Could you check a few things on this model? Use its own coordinates, in mm. Face numbers are marked on the shaded views. A direction names the side the tool comes from. Give positions to 0.01 mm unless a question says otherwise; leave off trailing zeros. Order: outer loops, then holes, each group sorted by start corner. A loop starts at its lowest first (then second) coordinate and runs counter-clockwise, first axis right, second up.
from build123d import *

# Parameters (mm, degrees)
SKETCH1_W           = 18
SKETCH1_H           = 14.75
BOSS_EXTRUDE1_DEPTH = 60
CUT_EXTRUDE1_REACH  = 123.108
SKETCH2_W           = 40
SKETCH2_H           = 14.75
CUT_EXTRUDE2_REACH  = 115.987
CUT_EXTRUDE3_REACH  = 123.108
SKETCH5_R           = 3.25
CUT_EXTRUDE4_REACH  = 105.817
SKETCH6_R           = 2.6
SKETCH7_R           = 2.6
CUT_EXTRUDE5_DEPTH  = 114.9871155
CUT_EXTRUDE6_REACH  = 115.987
SKETCH8_R           = 3.25
SKETCH9_W           = 23
SKETCH9_H           = 21.27
SKETCH9_H_2         = 20
CUT_EXTRUDE7_DEPTH  = 12
CHAMFER1_SIZE       = 1
CUT_EXTRUDE8_REACH  = 123.108
SKETCH10_R          = 3.1
SKETCH10_R_2        = 2.6
SKETCH11_R          = 3.25
CUT_EXTRUDE9_DEPTH  = 125.185596991
CHAMFER2_SIZE       = 1


with BuildPart() as part:
    # Sketch1 → Boss-Extrude1 (new body)
    with BuildSketch(Plane.XY):
        Polygon((0, 0), (-29, 0), (-29, 5), (-5, 5), (-5, 38), (-28, 38), (-28, 63.75), (-5, 63.75), (-5, 75.75), (18, 75.75), (18, 63.75), (73, 63.75), (73, 0), (52, 0), (52, 5), (68, 5), (68, 57.75), (0, 57.75), (0, 43), (18, 43), (18, 38), (0, 38), align=None)
        with Locations((-14, 50.375)):
            Rectangle(SKETCH1_W, SKETCH1_H, mode=Mode.SUBTRACT)
    extrude(amount=BOSS_EXTRUDE1_DEPTH)

    # Sketch2 → Cut-Extrude1 (cut, up to next)
    with BuildSketch(Plane(origin=(0, 0, 0), x_dir=(0, 0, -1), z_dir=(1, 0, 0)), mode=Mode.PRIVATE) as cut_extrude1_sk1:
        with Locations((-30, 51.375)):
            Rectangle(SKETCH2_W, SKETCH2_H)
    cut_extrude1_tool1 = extrude(cut_extrude1_sk1.sketch, amount=-CUT_EXTRUDE1_REACH, mode=Mode.PRIVATE) & part.part
    add(cut_extrude1_tool1.solids().sort_by_distance((0, 51.375, 30))[0], mode=Mode.SUBTRACT)

    # Sketch3 → Cut-Extrude2 (cut, up to next)
    with BuildSketch(Plane(origin=(0, 63.75, 0), x_dir=(1, 0, 0), z_dir=(0, 1, 0)), mode=Mode.PRIVATE) as cut_extrude2_sk1:
        with BuildLine():
            Line((39.5, -19), (46.5, -19))
            ThreePointArc((46.5, -19), (57.5, -30), (46.5, -41))
            Line((46.5, -41), (39.5, -41))
            ThreePointArc((39.5, -41), (28.5, -30), (39.5, -19))
        make_face()
    cut_extrude2_tool1 = extrude(cut_extrude2_sk1.sketch, amount=-CUT_EXTRUDE2_REACH, mode=Mode.PRIVATE) & part.part
    # Sketch3 → Cut-Extrude2 (cut, up to next)
    with BuildSketch(Plane(origin=(0, 63.75, 0), x_dir=(1, 0, 0), z_dir=(0, 1, 0)), mode=Mode.PRIVATE) as cut_extrude2_sk2:
        with BuildLine():
            Line((31, -16.1), (24, -16.1))
            ThreePointArc((24, -16.1), (22.4, -14.5), (24, -12.9))
            Line((24, -12.9), (31, -12.9))
            ThreePointArc((31, -12.9), (32.6, -14.5), (31, -16.1))
        make_face()
    cut_extrude2_tool2 = extrude(cut_extrude2_sk2.sketch, amount=-CUT_EXTRUDE2_REACH, mode=Mode.PRIVATE) & part.part
    # Sketch3 → Cut-Extrude2 (cut, up to next)
    with BuildSketch(Plane(origin=(0, 63.75, 0), x_dir=(1, 0, 0), z_dir=(0, 1, 0)), mode=Mode.PRIVATE) as cut_extrude2_sk3:
        with BuildLine():
            Line((55, -16.1), (62, -16.1))
            ThreePointArc((62, -16.1), (63.6, -14.5), (62, -12.9))
            Line((62, -12.9), (55, -12.9))
            ThreePointArc((55, -12.9), (53.4, -14.5), (55, -16.1))
        make_face()
    cut_extrude2_tool3 = extrude(cut_extrude2_sk3.sketch, amount=-CUT_EXTRUDE2_REACH, mode=Mode.PRIVATE) & part.part
    # Sketch3 → Cut-Extrude2 (cut, up to next)
    with BuildSketch(Plane(origin=(0, 63.75, 0), x_dir=(1, 0, 0), z_dir=(0, 1, 0)), mode=Mode.PRIVATE) as cut_extrude2_sk4:
        with BuildLine():
            Line((31, -43.9), (24, -43.9))
            ThreePointArc((24, -43.9), (22.4, -45.5), (24, -47.1))
            Line((24, -47.1), (31, -47.1))
            ThreePointArc((31, -47.1), (32.6, -45.5), (31, -43.9))
        make_face()
    cut_extrude2_tool4 = extrude(cut_extrude2_sk4.sketch, amount=-CUT_EXTRUDE2_REACH, mode=Mode.PRIVATE) & part.part
    # Sketch3 → Cut-Extrude2 (cut, up to next)
    with BuildSketch(Plane(origin=(0, 63.75, 0), x_dir=(1, 0, 0), z_dir=(0, 1, 0)), mode=Mode.PRIVATE) as cut_extrude2_sk5:
        with BuildLine():
            Line((55, -43.9), (62, -43.9))
            ThreePointArc((62, -43.9), (63.6, -45.5), (62, -47.1))
            Line((62, -47.1), (55, -47.1))
            ThreePointArc((55, -47.1), (53.4, -45.5), (55, -43.9))
        make_face()
    cut_extrude2_tool5 = extrude(cut_extrude2_sk5.sketch, amount=-CUT_EXTRUDE2_REACH, mode=Mode.PRIVATE) & part.part
    add(cut_extrude2_tool1.solids().sort_by_distance((43, 63.75, 30))[0], mode=Mode.SUBTRACT)
    add(cut_extrude2_tool2.solids().sort_by_distance((27.5, 63.75, 14.5))[0], mode=Mode.SUBTRACT)
    add(cut_extrude2_tool3.solids().sort_by_distance((58.5, 63.75, 14.5))[0], mode=Mode.SUBTRACT)
    add(cut_extrude2_tool4.solids().sort_by_distance((27.5, 63.75, 45.5))[0], mode=Mode.SUBTRACT)
    add(cut_extrude2_tool5.solids().sort_by_distance((58.5, 63.75, 45.5))[0], mode=Mode.SUBTRACT)

    # Sketch5 → Cut-Extrude3 (cut, up to next)
    with BuildSketch(Plane(origin=(0, 75.75, 0), x_dir=(1, 0, 0), z_dir=(0, 1, 0)), mode=Mode.PRIVATE) as cut_extrude3_sk1:
        with Locations(Location((9, -17.27, 0), (0, 0, 180))):
            Circle(SKETCH5_R)
    cut_extrude3_tool1 = extrude(cut_extrude3_sk1.sketch, amount=-CUT_EXTRUDE3_REACH, mode=Mode.PRIVATE) & part.part
    add(cut_extrude3_tool1.solids().sort_by_distance((9, 75.75, 17.27))[0], mode=Mode.SUBTRACT)

    # Sketch6 → Cut-Extrude4 (cut, up to next)
    with BuildSketch(Plane(origin=(0, 43, 0), x_dir=(1, 0, 0), z_dir=(0, 1, 0)), mode=Mode.PRIVATE) as cut_extrude4_sk1:
        with Locations(Location((9, -17.27, 0), (0, 0, 270))):
            Circle(SKETCH6_R)
    cut_extrude4_tool1 = extrude(cut_extrude4_sk1.sketch, amount=-CUT_EXTRUDE4_REACH, mode=Mode.PRIVATE) & part.part
    add(cut_extrude4_tool1.solids().sort_by_distance((9, 43, 17.27))[0], mode=Mode.SUBTRACT)

    # Sketch7 → Cut-Extrude5 (cut, through all)
    with BuildSketch(Plane(origin=(0, 63.75, 0), x_dir=(1, 0, 0), z_dir=(0, 1, 0))):
        with Locations(Location((-14, -30, 0), (0, 0, 270))):
            Circle(SKETCH7_R)
    extrude(amount=-CUT_EXTRUDE5_DEPTH, mode=Mode.SUBTRACT)

    # Sketch8 → Cut-Extrude6 (cut, up to next)
    with BuildSketch(Plane(origin=(0, 63.75, 0), x_dir=(1, 0, 0), z_dir=(0, 1, 0)), mode=Mode.PRIVATE) as cut_extrude6_sk1:
        with Locations(Location((-14, -30, 0), (0, 0, 270))):
            Circle(SKETCH8_R)
    cut_extrude6_tool1 = extrude(cut_extrude6_sk1.sketch, amount=-CUT_EXTRUDE6_REACH, mode=Mode.PRIVATE) & part.part
    add(cut_extrude6_tool1.solids().sort_by_distance((-14, 63.75, 30))[0], mode=Mode.SUBTRACT)

    # Sketch9 → Cut-Extrude7 (cut)
    with BuildSketch(Plane(origin=(0, 75.75, 0), x_dir=(1, 0, 0), z_dir=(0, 1, 0))):
        with Locations((6.5, -10.635)):
            Rectangle(SKETCH9_W, SKETCH9_H)
        with Locations((6.5, -50)):
            Rectangle(SKETCH9_W, SKETCH9_H_2)
    extrude(amount=-CUT_EXTRUDE7_DEPTH, mode=Mode.SUBTRACT)

    # Chamfer1
    # the kernel refuses this chamfer: 1 mm, written as the material it takes off along each edge
    with BuildSketch(Plane(origin=(-14, 63.75, 30), x_dir=(0, 0, 1), z_dir=(-1, 0, 0))) as chamfer1_piece_1:
        Polygon((3.25, -CHAMFER1_SIZE), (3.25 + CHAMFER1_SIZE, 0), (3.25, 0), align=None)
    revolve(axis=Axis((-14, 63.75, 30), (0, 1, 0)), mode=Mode.SUBTRACT)
    with BuildSketch(Plane(origin=(9, 63.75, 17.27), x_dir=(-1, 0, 0), z_dir=(0, 0, -1))) as chamfer1_piece_2_section:
        Polygon((3.25 + CHAMFER1_SIZE, 0), (3.25, -CHAMFER1_SIZE), (3.25, 0), align=None)
    chamfer1_piece_2 = revolve(axis=Axis((9, 63.75, 17.27), (0, 1, 0)), mode=Mode.PRIVATE)
    chamfer1_piece_2 = split(chamfer1_piece_2, bisect_by=Plane(origin=(12.733674615, 63.266325385, 21.27), z_dir=(0, 0, -1)), keep=Keep.TOP, mode=Mode.PRIVATE)
    add(chamfer1_piece_2, mode=Mode.SUBTRACT)

    # Sketch10 → Cut-Extrude8 (cut, up to next)
    with BuildSketch(Plane.XZ, mode=Mode.PRIVATE) as cut_extrude8_sk1:
        with Locations((-21, 45)):
            Circle(SKETCH10_R)
    cut_extrude8_tool1 = extrude(cut_extrude8_sk1.sketch, amount=-CUT_EXTRUDE8_REACH, mode=Mode.PRIVATE) & part.part
    # Sketch10 → Cut-Extrude8 (cut, up to next)
    with BuildSketch(Plane.XZ, mode=Mode.PRIVATE) as cut_extrude8_sk2:
        with Locations((-21, 15)):
            Circle(SKETCH10_R)
    cut_extrude8_tool2 = extrude(cut_extrude8_sk2.sketch, amount=-CUT_EXTRUDE8_REACH, mode=Mode.PRIVATE) & part.part
    # Sketch10 → Cut-Extrude8 (cut, up to next)
    with BuildSketch(Plane.XZ, mode=Mode.PRIVATE) as cut_extrude8_sk3:
        with Locations((60, 15)):
            Circle(SKETCH10_R_2)
    cut_extrude8_tool3 = extrude(cut_extrude8_sk3.sketch, amount=-CUT_EXTRUDE8_REACH, mode=Mode.PRIVATE) & part.part
    # Sketch10 → Cut-Extrude8 (cut, up to next)
    with BuildSketch(Plane.XZ, mode=Mode.PRIVATE) as cut_extrude8_sk4:
        with Locations((60, 45)):
            Circle(SKETCH10_R_2)
    cut_extrude8_tool4 = extrude(cut_extrude8_sk4.sketch, amount=-CUT_EXTRUDE8_REACH, mode=Mode.PRIVATE) & part.part
    add(cut_extrude8_tool1.solids().sort_by_distance((-21, 0, 45))[0], mode=Mode.SUBTRACT)
    add(cut_extrude8_tool2.solids().sort_by_distance((-21, 0, 15))[0], mode=Mode.SUBTRACT)
    add(cut_extrude8_tool3.solids().sort_by_distance((60, 0, 15))[0], mode=Mode.SUBTRACT)
    add(cut_extrude8_tool4.solids().sort_by_distance((60, 0, 45))[0], mode=Mode.SUBTRACT)

    # Sketch11 → Cut-Extrude9 (cut, through all)
    with BuildSketch(Plane.ZY.offset(5)):
        with Locations(Location((30.635, 69.75, 0), (0, 0, 270))):
            Circle(SKETCH11_R)
    extrude(amount=-CUT_EXTRUDE9_DEPTH, mode=Mode.SUBTRACT)

    # Chamfer2
    chamfer2_edges = [part.edges().sort_by_distance(p)[0] for p in [
        (-5, 73, 30.635),
    ]]
    chamfer(chamfer2_edges, length=CHAMFER2_SIZE)


solid = part.part
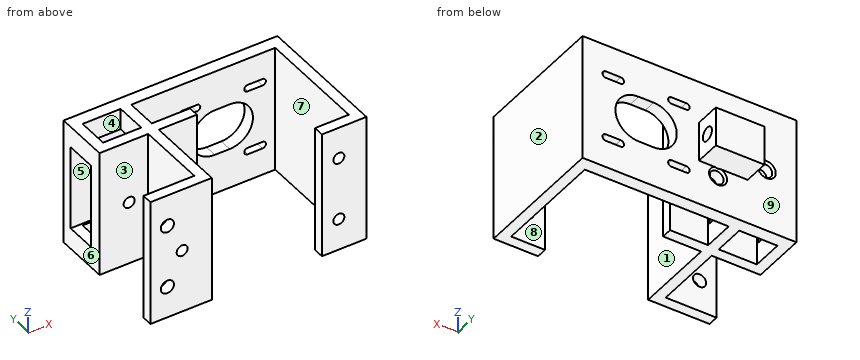
Item 1: Imagine slicing it at D-D on y = 14.5. List the corners of the cut face in (x, z) for me.
Findings:
outline: (-5, 0) - (0, 0) - (0, 60) - (-5, 60) - close; (68, 0) - (73, 0) - (73, 60) - (68, 60) - close
Item 2: Imagine slicing it at A-A on x = -21. List the corners of the cut face in (y, z) for me, then the cut area to 3 significant figures.
Findings:
outline: (0, 0) - (5, 0) - (5, 11.9) - (0, 11.9) - close; (0, 18.1) - (5, 18.1) - (5, 41.9) - (0, 41.9) - close; (0, 48.1) - (5, 48.1) - (5, 60) - (0, 60) - close; (38, 0) - (43, 0) - (43, 60) - (38, 60) - close; (57.75, 0) - (63.75, 0) - (63.75, 60) - (57.75, 60) - (57.75, 50) - (58.75, 50) - (58.75, 10) - (57.75, 10) - close
area: 858 mm2
Item 3: We'd pull the mould along X, two halves only. Please class the marked faces 6, 7, 8 and 9: +X half, -X half, draft (parallel to the pull), parting line (faces both ways), or undercut.
Findings:
face 6: -X half
face 7: undercut
face 8: undercut
face 9: draft
Item 4: For the marked faces 1, 2, 3, 4 and 5, which set-ups out of +Z, -Z, +X, -X, +Y, -Y let a thin tool reach every point of the face, with its end or its side?
Findings:
face 1: +Z, -Z, -Y
face 2: +Z, -Z, +X, +Y, -Y
face 3: +Z, -Z, -X
face 4: +Z, -Z
face 5: -X
Item 5: For pin 1 (8 mm diameter, centred on y = 50, z = 29.5, fed in from -X); pin 2 (19 mm diameter, centred on x = -16, z = 42.5, fed in from +Y); pin 3 (5.5 mm diameter, centred on x = -21, z = 15, fed in from -Y), each with a flat end and sliding along its axis, tell me the tip position at first contact or that it passes through.
Findings:
pin 1: stops at x = 68
pin 2: stops at y = 63.75
pin 3: stops at y = 38
Item 6: Please list where these lines run through material, in increasing order: line 1 along X through (y, z) = (61, 30); line 2 along Z through (x, y) = (-21, 1.4); line 3 along Y through (x, z) = (-16, 3).
Findings:
line 1: x = -28 to -17.25, -10.75 to 28.5, 57.5 to 73
line 2: z = 0 to 11.9, 18.1 to 41.9, 48.1 to 60
line 3: y = 0 to 5, 38 to 43, 57.75 to 63.75
Item 7: Imagine slicing it at C-C on y = 60.5. List the corners of the cut face in (x, z) for me, then the cut area to 3 significant figures.
Findings:
outline: (-28, 0) - (73, 0) - (73, 60) - (-28, 60) - close; hole circle Ø6.5 at (-14, 30); hole circle Ø6.5 at (9, 17.27); hole (24, 12.9) - (31, 12.9) arc R1.6 ccw to (31, 16.1) - (24, 16.1) arc R1.6 ccw to start; hole (24, 43.9) - (31, 43.9) arc R1.6 ccw to (31, 47.1) - (24, 47.1) arc R1.6 ccw to start; hole (39.5, 19) - (46.5, 19) arc R11 ccw to (46.5, 41) - (39.5, 41) arc R11 ccw to start; hole (55, 12.9) - (62, 12.9) arc R1.6 ccw to (62, 16.1) - (55, 16.1) arc R1.6 ccw to start; hole (55, 43.9) - (62, 43.9) arc R1.6 ccw to (62, 47.1) - (55, 47.1) arc R1.6 ccw to start
area: 5,340 mm2
Item 8: Imagine slicing it at B-B on y = 45.5. List the corners of the cut face in (x, z) for me, then the cut area to 3 significant figures.
Findings:
outline: (-28, 0) - (-23, 0) - (-23, 10) - (-28, 10) - close; (-28, 50) - (-23, 50) - (-23, 60) - (-28, 60) - close; (-5, 0) - (0, 0) - (0, 10) - (-5, 10) - close; (-5, 50) - (0, 50) - (0, 60) - (-5, 60) - close; (68, 0) - (73, 0) - (73, 60) - (68, 60) - close
area: 500 mm2
